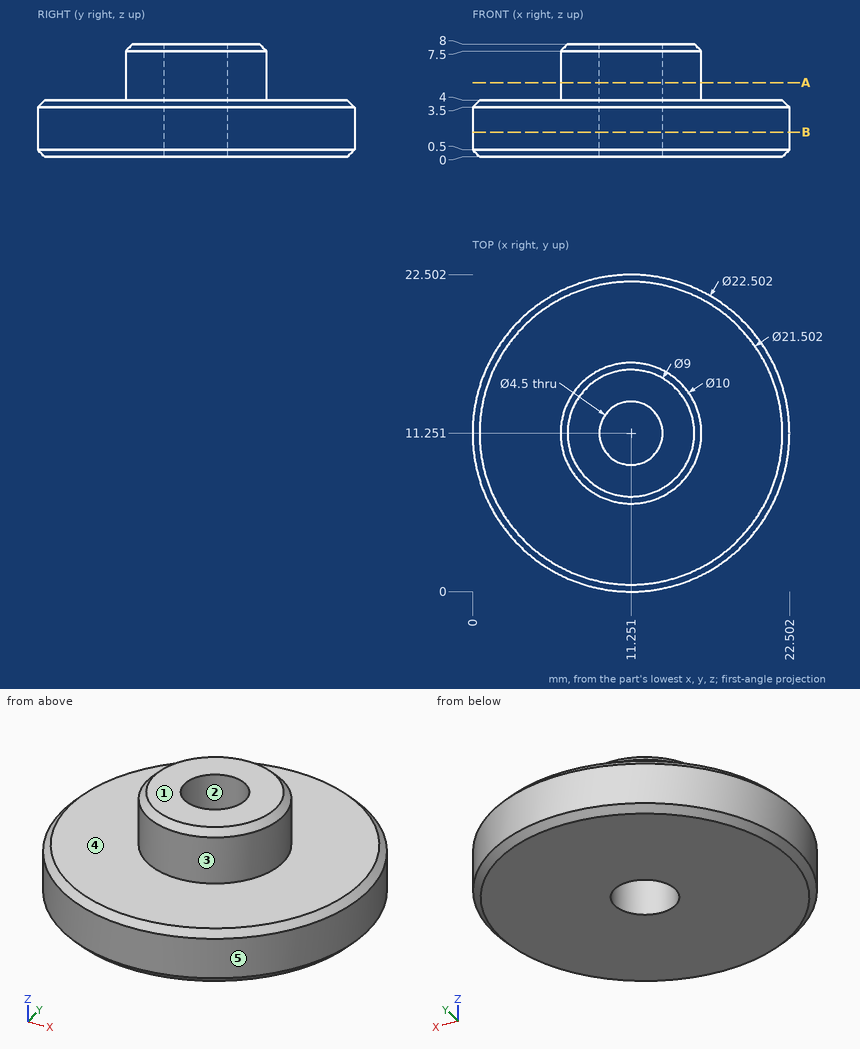
Input: dimensioned drawing with shaded views. Units: mm. Origin: part minimum x, y, z. A direction names the side the tool comes from. Round coordinates to 2 decimals unless told otherwise and drop trailing zeros. Order: outer loops, then holes, each group sorted by start corner. A loop starts at its lowest first (then second) coordinate and runs counter-clockwise, first axis right, second up. Notation, with made-up numbers: (82.25, -30) - (89.25, -30) arc R28 ccw to (89.25, -9) - close; hole circle Ø8 at (-30.5, 24.25). An arc over 180 degrees is marked (long way). Answer as a JSON object with one key per item and string values. Group by question number.
(1) Reachability of the marked faces 4 and 5 from +Z, -Z, +X, -X, +Y, -Y: full face, straight path, thin tool, end or side. Return the list, or none.
(2) Draft query along X for the marked faces 1, 2 and 3. Return one class per face: released by +X, released by -X, zero draft, split by the parting line, or undercut.
(3) Pin query (flat end, axial travel): P1, Ø3, axis at y = 5, z = 1.5, coming from the +X side; P2, Ø3, axis at y = 6, z = 7, coming from the +X side; P3, Ø1.5, axis at x = 13.5, z = 3, coming from the -Y side. Return the tip coordinate at first contact, or that it passes through.
(4) Material intervals for probe 1 along Z at (x, y) = (17.5, 15.75); probe 2 along Y at (x, z) = (12, 5.75); probe 3 along X at (y, z) = (12.75, 7), sorted ascending. Write a range as from..to.
(5) Cut plane A-A (z = 5.25). Return loops of the section in (x, y).
(6) Cut plane B-B (z = 1.75). Return loops of the section in (x, y), then the cut area to 3 significant figures.
Here are the results:
{
 "1": {"face 4": "+Z", "face 5": "+Z, -Z"},
 "2": {"face 1": "zero draft", "face 2": "undercut", "face 3": "split by the parting line"},
 "3": {"P1": "stops at x = 21.45", "P2": "stops at x = 14.56", "P3": "stops at y = 0.1"},
 "4": {"probe 1": "z = 0..4", "probe 2": "y = 6.31..9.13, 13.37..16.19", "probe 3": "x = 6.48..9.57, 12.93..16.02"},
 "5": {"outline": "circle Ø10 at (11.25, 11.25); hole circle Ø4.5 at (11.25, 11.25)"},
 "6": {"outline": "circle Ø22.5 at (11.25, 11.25); hole circle Ø4.5 at (11.25, 11.25)", "area": "382 mm^2"}
}
